Can you work these out from the model? Positions are in its coordinate system, mm. A direction names the side the tool comes from. Give positions to 0.01 mm unless a question says otherwise; leave off trailing zeros. Loops run counter-clockwise (first coordinate to the right, second up) from the corner with the lowest first, then second, coordinate; pieces in that order, holes last. Notation, with made-up numbers: (-15.75, 81.25) - (1.25, 81.25) arc R27 ccw to (1.25, 112.25) - close; hole circle Ø11 at (51, -7.75). An arc over 180 degrees is marked (long way). Write item = value, one per line.
from build123d import *

# Parameters (mm, degrees)
SKETCH1_W                     = 101.6
SKETCH1_H                     = 63.5
BOSS_EXTRUDE1_DEPTH           = 57.15
CBORE_FOR_M3_SHCS1_AT_2_COUNT = 2
CBORE_FOR_M3_SHCS1_AT_2_PITCH = 15.499969
CBORE_FOR_M3_SHCS1_AT_3_COUNT = 2
CBORE_FOR_M3_SHCS1_AT_3_PITCH = 26.846733824
CBORE_FOR_M3_SHCS1_AT_4_COUNT = 2
CBORE_FOR_M3_SHCS1_AT_4_PITCH = 30.999938
CBORE_FOR_M3_SHCS1_AT_5_COUNT = 2
CBORE_FOR_M3_SHCS1_AT_5_PITCH = 26.846733824
CBORE_FOR_M3_SHCS1_AT_6_COUNT = 2
CBORE_FOR_M3_SHCS1_AT_6_PITCH = 15.499969
SKETCH8_R                     = 6.223
CUT_EXTRUDE1_DEPTH            = 50.8
SKETCH9_W                     = 76.2
SKETCH9_H                     = 50.8
CUT_EXTRUDE2_DEPTH            = 53.34
CUT_EXTRUDE3_START            = -19.05
SKETCH2_R                     = 18.542
CUT_EXTRUDE3_DEPTH            = 13.97
SKETCH10_W                    = 101.6
SKETCH10_H                    = 12.7
BOSS_EXTRUDE2_DEPTH           = 3.81
CUT_EXTRUDE4_DEPTH            = 3.81


with BuildPart() as part:
    # Sketch1 → Boss-Extrude1 (new body)
    with BuildSketch(Plane(origin=(0, 0, 0), x_dir=(1, 0, 0), z_dir=(0, 1, 0))):
        Rectangle(SKETCH1_W, SKETCH1_H)
    extrude(amount=BOSS_EXTRUDE1_DEPTH)

    # Sketch6 → CBORE for M3 SHCS1 (revolve, cut)
    with BuildSketch(Plane(origin=(50.8, 41.998366912, 7.7499845), x_dir=(0, 0, -1), z_dir=(0, 1, 0))):
        Polygon((0, 0), (0, 6.101463052), (1.7, 5.08), (1.7, 3), (3.25, 3), (3.25, 0.025), (3.275, 0), align=None)
    cbore_for_m3_shcs1 = revolve(axis=Axis((57.15, 41.998366912, 7.7499845), (-1, 0, 0)), mode=Mode.SUBTRACT)

    # CBORE for M3 SHCS1 at 2: CBORE for M3 SHCS1 ×2
    with Locations(*[Vector(0, -0.866025404, 0.5) * (i * CBORE_FOR_M3_SHCS1_AT_2_PITCH) for i in range(1, CBORE_FOR_M3_SHCS1_AT_2_COUNT)]):
        add(cbore_for_m3_shcs1, mode=Mode.SUBTRACT)

    # CBORE for M3 SHCS1 at 3: CBORE for M3 SHCS1 ×2
    with Locations(*[(0, -i * CBORE_FOR_M3_SHCS1_AT_3_PITCH, 0) for i in range(1, CBORE_FOR_M3_SHCS1_AT_3_COUNT)]):
        add(cbore_for_m3_shcs1, mode=Mode.SUBTRACT)

    # CBORE for M3 SHCS1 at 4: CBORE for M3 SHCS1 ×2
    with Locations(*[Vector(0, -0.866025404, -0.5) * (i * CBORE_FOR_M3_SHCS1_AT_4_PITCH) for i in range(1, CBORE_FOR_M3_SHCS1_AT_4_COUNT)]):
        add(cbore_for_m3_shcs1, mode=Mode.SUBTRACT)

    # CBORE for M3 SHCS1 at 5: CBORE for M3 SHCS1 ×2
    with Locations(*[Vector(0, -0.5, -0.866025404) * (i * CBORE_FOR_M3_SHCS1_AT_5_PITCH) for i in range(1, CBORE_FOR_M3_SHCS1_AT_5_COUNT)]):
        add(cbore_for_m3_shcs1, mode=Mode.SUBTRACT)

    # CBORE for M3 SHCS1 at 6: CBORE for M3 SHCS1 ×2
    with Locations(*[(0, 0, -i * CBORE_FOR_M3_SHCS1_AT_6_PITCH) for i in range(1, CBORE_FOR_M3_SHCS1_AT_6_COUNT)]):
        add(cbore_for_m3_shcs1, mode=Mode.SUBTRACT)

    # Sketch8 → Cut-Extrude1 (cut)
    with BuildSketch(Plane(origin=(50.8, 29.820388237, 44.133609073), x_dir=(0, 0, 1), z_dir=(1, 0, 0))):
        with Locations((-44.133609073, 8.245386937)):
            Circle(SKETCH8_R)
    extrude(amount=-CUT_EXTRUDE1_DEPTH, mode=Mode.SUBTRACT)

    # Sketch9 → Cut-Extrude2 (cut)
    with BuildSketch(Plane(origin=(0, 57.15, 0), x_dir=(1, 0, 0), z_dir=(0, 1, 0))):
        with Locations((-6.35, 0)):
            Rectangle(SKETCH9_W, SKETCH9_H)
    extrude(amount=-CUT_EXTRUDE2_DEPTH, mode=Mode.SUBTRACT)

    # Sketch2 → Cut-Extrude3 (cut)
    with BuildSketch(Plane(origin=(50.8, 29.820388237, 50.894246884), x_dir=(0, 0, -1), z_dir=(1, 0, 0)).offset(CUT_EXTRUDE3_START)):
        with Locations((50.894246884, -1.245388237)):
            Circle(SKETCH2_R)
    extrude(amount=CUT_EXTRUDE3_DEPTH, mode=Mode.SUBTRACT)

    # Sketch10 → Boss-Extrude2 (add)
    with BuildSketch(Plane(origin=(0, 57.15, 0), x_dir=(1, 0, 0), z_dir=(0, 1, 0))):
        with Locations((0, 38.1)):
            Rectangle(SKETCH10_W, SKETCH10_H)
        with Locations((0, -38.1)):
            Rectangle(SKETCH10_W, SKETCH10_H)
    extrude(amount=-BOSS_EXTRUDE2_DEPTH)

    # Sketch11 → Cut-Extrude4 (cut)
    with BuildSketch(Plane(origin=(0, 57.15, 0), x_dir=(1, 0, 0), z_dir=(0, 1, 0))):
        with BuildLine():
            Line((-44.45, 39.8018), (44.45, 39.8018))
            ThreePointArc((44.45, 39.8018), (46.1518, 38.1), (44.45, 36.3982))
            Line((44.45, 36.3982), (-44.45, 36.3982))
            ThreePointArc((-44.45, 36.3982), (-46.1518, 38.1), (-44.45, 39.8018))
        make_face()
        with BuildLine():
            Line((-44.45, -39.8018), (44.45, -39.8018))
            ThreePointArc((44.45, -39.8018), (46.1518, -38.1), (44.45, -36.3982))
            Line((44.45, -36.3982), (-44.45, -36.3982))
            ThreePointArc((-44.45, -36.3982), (-46.1518, -38.1), (-44.45, -39.8018))
        make_face()
    extrude(amount=-CUT_EXTRUDE4_DEPTH, mode=Mode.SUBTRACT)


solid = part.part
Q1. Imagine slicing it at C-C, the plane y = 8. Write out the boundary of the cut face in (x, z).
Output:
outline = (-50.8, -31.75) - (50.8, -31.75) - (50.8, 31.75) - (-50.8, 31.75) - close; hole (-44.45, -25.4) - (31.75, -25.4) - (31.75, 25.4) - (-44.45, 25.4) - close
Q2. We'd pull the mould along X, two halves only. Please class faces 5 (the cylindrical face through (-46.15, 55.27, 38.06)), 6 (the cylindrical face through (48.296, 15.405, -0.81)), 7 (the flat face through (-50.8, 29, 1)): released by +X, released by -X, zero draft, split by the parting line, or undercut.
Output:
face_5 = undercut
face_6 = zero draft
face_7 = released by -X
Q3. For pin 1 (4 mm diameter, centred on y = 15.15, z = 7.75, fed in from +X); pin 2 (4 mm diameter, centred on x = -38, y = 50, fed in from +Z); pin 3 (7 mm diameter, centred on y = 28.5, z = 14, fed in from +X); pin 4 (2 mm diameter, centred on x = 7.5, y = 51.5, fed in from -Z), each with a flat end and sliding along its axis, tell me the tip position at first contact or that it passes through.
Output:
pin_1 = 47.8
pin_2 = 31.75
pin_3 = 50.8
pin_4 = -31.75
Q4. Which directions (+Z, -Z, +X, -X, +Y, -Y) give clear straight access to the entire face, cutting with the end or side of a thin tool? Please do faces 1 (the flat face through (31.75, 49, 0)), 2 (the flat face through (-1, 53.34, 35)), 3 (the flat face through (45.72, 29, 0)), 4 (the cylindrical face through (49.31, 31.75, 16.2)).
Output:
face_1 = +Y
face_2 = +Z, +X, -X, -Y
face_3 = none
face_4 = +X
Q5. Imagine slicing it at D-D, the plane z = 0. Write out the boundary of the cut face in (x, y), then the cut area to 3 significant figures.
Output:
outline = (-50.8, 0) - (50.8, 0) - (50.8, 15.35) - (45.72, 15.35) - (45.72, 10.03) - (31.75, 10.03) - (31.75, 3.81) - (-44.45, 3.81) - (-44.45, 57.15) - (-50.8, 57.15) - close; (31.75, 47.12) - (45.72, 47.12) - (45.72, 27.8) - (50.8, 27.8) - (50.8, 57.15) - (31.75, 57.15) - close
area = 1,160 mm2
Q6. Imagine slicing it at A-A, the plane z = -38.1. Write out the boundary of the cut face in (x, y), then the cut area to 3 significant figures.
Output:
outline = (-50.8, 53.34) - (-46.15, 53.34) - (-46.15, 57.15) - (-50.8, 57.15) - close; (46.15, 53.34) - (50.8, 53.34) - (50.8, 57.15) - (46.15, 57.15) - close
area = 35.4 mm2
Q7. Imagine slicing it at B-B, the plane x = -23.5. Write out the boundary of the cut face in (y, z), then the cut area to 3 significant figures.
Output:
outline = (0, -31.75) - (53.34, -31.75) - (53.34, -36.4) - (57.15, -36.4) - (57.15, -25.4) - (3.81, -25.4) - (3.81, 25.4) - (57.15, 25.4) - (57.15, 36.4) - (53.34, 36.4) - (53.34, 31.75) - (0, 31.75) - close; (53.34, -44.45) - (57.15, -44.45) - (57.15, -39.8) - (53.34, -39.8) - close; (53.34, 39.8) - (57.15, 39.8) - (57.15, 44.45) - (53.34, 44.45) - close
area = 990 mm2
Q8. I need wall thicknesses on L1, parallel to Z at x = -16, y = 6.5; L2, parallel to X at y = 26.5, z = 24; L3, parallel to X at y = 27.5, z = -13.5. Which ranges of each line are inside material? Lowest first, please.
Output:
L1 = -31.75 to -25.4, 25.4 to 31.75
L2 = -50.8 to -44.45, 31.75 to 50.8
L3 = -50.8 to -44.45, 45.72 to 47.8
